from build123d import *

# Parameters (mm, degrees)
SKETCH1_W           = 16
SKETCH1_H           = 16
BOSS_EXTRUDE1_DEPTH = 11
FILLET1_R           = 1
SKETCH4_R           = 3
BOSS_EXTRUDE2_DEPTH = 4
BOSS_EXTRUDE3_DEPTH = 2
SKETCH3_R           = 2.715
CUT_EXTRUDE2_DEPTH  = 22.106870919
CUT_EXTRUDE3_DEPTH  = 20.735754356


with BuildPart() as part:
    # Sketch1 → Boss-Extrude1 (new body)
    with BuildSketch(Plane(origin=(0, 0, 0), x_dir=(1, 0, 0), z_dir=(0, 1, 0))):
        Rectangle(SKETCH1_W, SKETCH1_H)
    extrude(amount=BOSS_EXTRUDE1_DEPTH)

    # Fillet1
    fillet1_edges = [part.edges().sort_by_distance(p)[0] for p in [
        (8, 5.5, 8),
        (-8, 5.5, 8),
        (-8, 5.5, -8),
        (8, 5.5, -8),
    ]]
    fillet(fillet1_edges, radius=FILLET1_R)

    # Sketch4 → Boss-Extrude2 (add)
    with BuildSketch(Plane(origin=(0, 0, 0), x_dir=(-1, 0, 0), z_dir=(0, -1, 0))):
        with Locations(Location((3.5, 0, 0), (0, 0, 90))):
            Circle(SKETCH4_R)
        with Locations(Location((-3.5, 0, 0), (0, 0, 90))):
            Circle(SKETCH4_R)
    extrude(amount=BOSS_EXTRUDE2_DEPTH)

    # Sketch5 → Boss-Extrude3 (add)
    with BuildSketch(Plane(origin=(0, -4, 0), x_dir=(-1, 0, 0), z_dir=(0, -1, 0))):
        with BuildLine():
            Line((9.5, 10.5), (-9.5, 10.5))
            ThreePointArc((-9.5, 10.5), (-10.207106781, 10.207106781), (-10.5, 9.5))
            Line((-10.5, 9.5), (-10.5, -9.5))
            ThreePointArc((-10.5, -9.5), (-10.207106781, -10.207106781), (-9.5, -10.5))
            Line((-9.5, -10.5), (9.5, -10.5))
            ThreePointArc((9.5, -10.5), (10.207106781, -10.207106781), (10.5, -9.5))
            Line((10.5, -9.5), (10.5, 9.5))
            ThreePointArc((10.5, 9.5), (10.207106781, 10.207106781), (9.5, 10.5))
        make_face()
    extrude(amount=-BOSS_EXTRUDE3_DEPTH)

    # Sketch3 → Cut-Extrude2 (cut, through all)
    with BuildSketch(Plane(origin=(0, 11, 0), x_dir=(1, 0, 0), z_dir=(0, 1, 0))):
        with Locations(Location((-3.5, 0, 0), (0, 0, 270))):
            Circle(SKETCH3_R)
        with Locations(Location((3.5, 0, 0), (0, 0, 270))):
            Circle(SKETCH3_R)
    extrude(amount=-CUT_EXTRUDE2_DEPTH, mode=Mode.SUBTRACT)

    # Sketch7 → Cut-Extrude3 (cut, through all)
    with BuildSketch(Plane(origin=(0, -2, 0), x_dir=(1, 0, 0), z_dir=(0, 1, 0))):
        with BuildLine():
            Line((0, -9.085786438), (1.414213562, -10.5))
            Line((1.414213562, -10.5), (3.889087297, -8.025126266))
            ThreePointArc((3.889087297, -8.025126266), (4.035533906, -7.671572875), (3.889087297, -7.318019485))
            Line((3.889087297, -7.318019485), (3.181980515, -6.610912703))
            ThreePointArc((3.181980515, -6.610912703), (2.828427125, -6.464466094), (2.474873734, -6.610912703))
            Line((2.474873734, -6.610912703), (0, -9.085786438))
        make_face()
        with BuildLine():
            Line((-3.889087297, -8.025126266), (-1.414213562, -10.5))
            Line((-1.414213562, -10.5), (0, -9.085786438))
            Line((0, -9.085786438), (-2.474873734, -6.610912703))
            ThreePointArc((-2.474873734, -6.610912703), (-2.828427125, -6.464466094), (-3.181980515, -6.610912703))
            Line((-3.181980515, -6.610912703), (-3.889087297, -7.318019485))
            ThreePointArc((-3.889087297, -7.318019485), (-4.035533906, -7.671572875), (-3.889087297, -8.025126266))
        make_face()
        Polygon((-1.414213562, -10.5), (1.414213562, -10.5), (0, -9.085786438), align=None)
    extrude(amount=-CUT_EXTRUDE3_DEPTH, mode=Mode.SUBTRACT)


solid = part.part
Design review of the part built by this model. Coordinates are the model's own, in mm. A direction names the side the tool comes from. Give positions to 0.01 mm unless a question says otherwise; leave off trailing zeros. Order: outer loops, then holes, each group sorted by start corner. A loop starts at its lowest first (then second) coordinate and runs counter-clockwise, first axis right, second up. Notation, with made-up numbers: (20, 36.5) - (25, 36.5) arc R31 cw to (25, 71.5) - close; hole circle Ø10 at (-24.5, -39). An arc over 180 degrees is marked (long way). Use CSV: the item, a comma, the result in double quotes. Start each with the question number.
Q1. Take a section at D-D (z = -6.25). State the section outline as (x, y) points, and give its area (3 significant figures).
Q2. Take a section at B-B (y = -2.75). State the section outline as (x, z) points (3 decimals).
Q3. Take a section at A-A (z = 0). State the section outline as (x, y) points (3 decimals).
Q4. For P1, Ø3.5, axis at x = 0.5, y = 8, coming from the +Z side; P2, Ø8, axis at y = 7.5, z = -5, coming from the -X side; P3, Ø2, axis at y = 4, z = 2.5, coming from the +X side, all flat-tipped, find the tip position at first contact; note any pin that passes through.
Q5. Take a section at C-C (x = 3.5). State the section outline as (y, z) points (3 decimals).
Q6. Machinability: for faces 5 (the face through (-1.22, -2.986, 7.866)), 6 (the face through (-8, 5, 0)), 7 (the face through (-7.715, 5.577, 7.699)), 8 (the face through (7.715, 5.577, -7.699)), which of the approach directions +Z, -Z, +X, -X, +Y, -Y give a long, thin tool a straight path to every point of the face, cutting with its end or side? Answer none if there is none.
Q7. Draft analysis for pull direction Z (two halves, no side actions). For faces 1 (the face through (10.215, -3.014, 10.199)), 2 (the face through (-1.21, 3.61, 1.46)), 3 (the face through (0, -2, 0)), 4 (the face through (0, 5, -8)), state which applies: pulls with the +Z half, pulls with the -Z half, needs draft (parallel to the pull), parting line crosses it, or undercut.
Q8. For line 1 (X direction, y = 4.5, z = 0) (3 decimals); line 2 (Y direction, x = -6.5, z = 2.5); line 3 (X direction, y = 4, z = 1), list the stretches that pass through material, from the lowest coordinate up.
Calculated:
1,outline,"(-10.5, -4) - (10.5, -4) - (10.5, -2) - (-10.5, -2) - close; (-8, 0) - (8, 0) - (8, 11) - (-8, 11) - close"
1,area,"218 mm²"
2,outline,"(-10.5, -9.5) arc R1 ccw to (-9.5, -10.5) - (9.5, -10.5) arc R1 ccw to (10.5, -9.5) - (10.5, 9.5) arc R1 ccw to (9.5, 10.5) - (1.414, 10.5) - (3.889, 8.025) arc R0.5 cw to (3.889, 7.318) - (3.182, 6.611) arc R0.5 cw to (2.475, 6.611) - (0, 9.086) - (-2.475, 6.611) arc R0.5 cw to (-3.182, 6.611) - (-3.889, 7.318) arc R0.5 cw to (-3.889, 8.025) - (-1.414, 10.5) - (-9.5, 10.5) arc R1 ccw to (-10.5, 9.5) - close; hole circle Ø5.43 at (-3.5, 0); hole circle Ø5.43 at (3.5, 0)"
3,outline,"(-10.5, -4) - (-6.215, -4) - (-6.215, 11) - (-8, 11) - (-8, 0) - (-6.5, 0) - (-6.5, -2) - (-10.5, -2) - close; (-0.785, -4) - (0.785, -4) - (0.785, 11) - (-0.785, 11) - close; (6.215, -4) - (10.5, -4) - (10.5, -2) - (6.5, -2) - (6.5, 0) - (8, 0) - (8, 11) - (6.215, 11) - close; hole (-0.5, -2) - (0.5, -2) - (0.5, 0) - (-0.5, 0) - close"
4,P1,"stops at z = 8"
4,P2,"stops at x = -8"
4,P3,"stops at x = 8"
5,outline,"(-4, -10.5) - (-2, -10.5) - (-2, -3) - (0, -3) - (0, -8) - (11, -8) - (11, -2.715) - (-4, -2.715) - close; (-4, 2.715) - (11, 2.715) - (11, 8) - (0, 8) - (0, 3) - (-2, 3) - (-2, 6.929) - (-4, 6.929) - close; (-4, 8.414) - (-2, 8.414) - (-2, 10.5) - (-4, 10.5) - close"
6,face 5,"-Y"
6,face 6,"+Z, -Z, -X, +Y"
6,face 7,"+Z, -X, +Y"
6,face 8,"-Z, +X, +Y"
7,face 1,"pulls with the +Z half"
7,face 2,"undercut"
7,face 3,"needs draft"
7,face 4,"pulls with the -Z half"
8,line 1,"x = -8 to -6.215, -0.785 to 0.785, 6.215 to 8"
8,line 2,"y = -4 to -2, 0 to 11"
8,line 3,"x = -8 to -6.02, -0.98 to 0.98, 6.02 to 8"
